```python
from build123d import *

# Parameters (mm, degrees)
F1_DEPTH = 10
F2_R     = 8
F3_DEPTH = 35
F4_SIZE  = 1.5


with BuildPart() as f1:
    # F0 (on Top) → F1 (new body)
    with BuildSketch(Plane.XY):
        Polygon((12, -6.928203), (12, 6.928203), (0, 13.856406), (-12, 6.928203), (-12, -6.928203), (0, -13.856406), align=None)
    extrude(amount=F1_DEPTH)

    # F2 (on face) → F3 (join)
    with BuildSketch(Plane.XY.offset(10)):
        Circle(F2_R)
    extrude(amount=F3_DEPTH)

    # F4
    f4_edges = [f1.edges().sort_by_distance(p)[0] for p in [
        (-8, 0, 45),
    ]]
    chamfer(f4_edges, length=F4_SIZE)


solid = f1.part
```
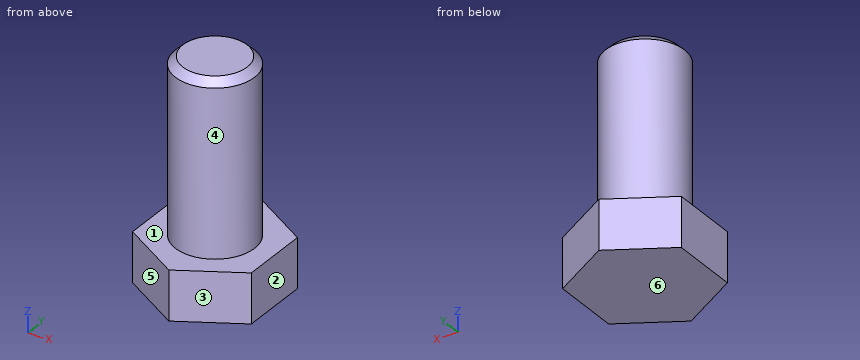
For this review, take the finished solid that the model builds, in its own axes (mm). Face numbers are marked on the shaded views. A direction names the side the tool comes from. Round coordinates to 2 decimals unless told otherwise and drop trailing zeros. Write each loop counter-clockwise with the first axis right and the second up, starting at its lowest first coordinate (ties: lowest second). Pieces come first, ordered by that corner, then holes. Notation, with made-up numbers: (-5, -23) - (52, -23) arc R14 ccw to (52, -6) - close; hole circle Ø5 at (41.25, 74). An arc over 180 degrees is marked (long way). Answer as a JSON object with one key per item and string values.
1. We need section C-C on x = -10.25. Give the boundary of the cut face in (y, z), then the cut area to 3 significant figures.
Response values:
{"outline": "(-7.94, 0) - (7.94, 0) - (7.94, 10) - (-7.94, 10) - close", "area": "159 mm2"}
2. For pin 1 Ø6 at (y, z) = (3, 22) entering from +X; pin 2 Ø1 at (x, z) = (2, 16) entering from +Y; pin 3 Ø4 at (x, z) = (8, 18.5) entering from +Y, all flat-tipped, find the tip position at first contact; note any pin that passes through.
Response values:
{"pin 1": "stops at x = 8", "pin 2": "stops at y = 7.86", "pin 3": "stops at y = 5.29"}
3. We need section A-A on y = 0. Give the boundary of the cut face in (x, z), then the cut area to 3 significant figures.
Response values:
{"outline": "(-12, 0) - (12, 0) - (12, 10) - (8, 10) - (8, 43.5) - (6.5, 45) - (-6.5, 45) - (-8, 43.5) - (-8, 10) - (-12, 10) - close", "area": "798 mm2"}
4. To check wall thickness, follow line 1 along Z through (x, y) = (4.25, 10.5); line 2 along X through (y, z) = (-4.5, 30.5); line 3 along Y through (x, z) = (7.25, 6.5). State the ranges of each line that lie inside material, in increasing order.
Response values:
{"line 1": "z = 0 to 10", "line 2": "x = -6.61 to 6.61", "line 3": "y = -9.67 to 9.67"}
5. Draft analysis for pull direction X (two halves, no side actions). For the marked faces 3, 4, 5 and 6, state which applies: +X half, -X half, draft (parallel to the pull), parting line (faces both ways), or undercut.
Response values:
{"face 3": "+X half", "face 4": "parting line", "face 5": "-X half", "face 6": "draft"}
6. Tool access review of the marked faces 1 and 2: name each direction out of +Z, -Z, +X, -X, +Y, -Y from which nothing blocks a thin tool from reaching the whole face with its end or side.
Response values:
{"face 1": "+Z", "face 2": "+Z, -Z, +X, +Y, -Y"}
7. We need section D-D on z = 18. Give the boundary of the cut face in (x, y).
Response values:
{"outline": "circle Ø16 at (0, 0)"}
8. We need section B-B on z = 5. Give the boundary of the cut face in (x, y).
Response values:
{"outline": "(-12, -6.93) - (0, -13.86) - (12, -6.93) - (12, 6.93) - (0, 13.86) - (-12, 6.93) - close"}
